Model file for the job. Use its own axes, mm. A direction names the side the tool comes from. Coordinates: 2 decimals unless noted, no trailing zeros. Loops run counter-clockwise (first coordinate to the right, second up) from the corner with the lowest first, then second, coordinate; pieces in that order, holes last. Notation, with made-up numbers: (57, -5.75) -> (90, -5.75) arc R17 cw to (90, 22.25) -> close; hole circle Ø6 at (-13.5, -22.5). An arc over 180 degrees is marked (long way). Use one line per item in the form item = value.
```python
from build123d import *

# Parameters (mm, degrees)
F0_W     = 48.26
F0_H     = 30.48
F0_W_2   = 45.72
F0_H_2   = 27.94
F1_DEPTH = 17.78
F2_DEPTH = 1.27
F3_R     = 7.62
F5_W     = 48.26
F5_H     = 17.78
F6_DEPTH = 1.27
F4_R     = 8.001
F4_R_2   = 7.62
F7_DEPTH = 12.1666


with BuildPart() as f1:
    # F0 (on Top) → F1 (new body)
    with BuildSketch(Plane.XY):
        with Locations((-40.818777, 0.441459)):
            Rectangle(F0_W, F0_H)
        with Locations((-40.818777, 0.441459)):
            Rectangle(F0_W_2, F0_H_2, mode=Mode.SUBTRACT)
    extrude(amount=F1_DEPTH)

    # F0 (on Top) → F2 (join)
    with BuildSketch(Plane.XY):
        with Locations((-40.818777, 0.441459)):
            Rectangle(F0_W_2, F0_H_2)
    extrude(amount=F2_DEPTH)

    # F3
    f3_edges = [f1.edges().sort_by_distance(p)[0] for p in [
        (-16.688777, 15.681459, 8.89),
        (-17.958777, 14.411459, 9.525),
    ]]
    fillet(f3_edges, radius=F3_R)

    # F5 (on face) → F6 (cut)
    with BuildSketch(Plane.XZ.offset(14.798541)):
        with Locations((-40.818777, 8.89)):
            Rectangle(F5_W, F5_H)
    extrude(amount=-F6_DEPTH, mode=Mode.SUBTRACT)

    # F4 (on face) → F7 (cut)
    with BuildSketch(Plane.XY.offset(1.27)):
        with Locations((-40.818777, 0.441459)):
            Circle(F4_R)
        with Locations((-26.086777, 6.283459)):
            Circle(F4_R_2)
        with Locations((-55.550777, -5.400541)):
            Circle(F4_R_2)
    extrude(amount=-F7_DEPTH, mode=Mode.SUBTRACT)


solid = f1.part
```
Q1. Which spindle directions (+Z, -Z, +X, -X, +Y, -Y) get a long thin tool onto all of the face, cutting with end or side? Do faces 1 (the face through (-41, 15, 17.78)), 2 (the face through (-17.959, -4, 9)). Say none if no direction does.
Result:
face_1 = +Z, +X, -X, +Y, -Y
face_2 = +Z, -Y
Q2. Mould opens along X. For faces 3 (the face through (-46, -6, 1.27)), 4 (the face through (-16.689, -3, 9)), 5 (the face through (-47, 8, 0)) say: released by +X, released by -X, zero draft, split by the parting line, or undercut.
Result:
face_3 = undercut
face_4 = released by +X
face_5 = zero draft
Q3. Pin check, flat tips, straight feed: pin 1 Ø8 at (x, y) = (-37, 7.5) entering from +Z; pin 2 Ø4 at (x, y) = (-29.5, 8) entering from -Z; pin 3 Ø4 at (x, z) = (-24.5, 11.5) entering from -Y. Stop position of each tip, or through.
Result:
pin_1 = 1.27
pin_2 = through
pin_3 = 13.76
Q4. Band-saw the part on A-A, the plane x = -53. Write the cut outline in (y, z), and give its area (3 significant figures).
Result:
outline = (-13.53, 0) -> (-12.58, 0) -> (-12.58, 1.27) -> (-13.53, 1.27) -> close; (1.78, 0) -> (15.68, 0) -> (15.68, 17.78) -> (14.41, 17.78) -> (14.41, 1.27) -> (1.78, 1.27) -> close
area = 39.8 mm2
Q5. Band-saw the part on B-B, the plane y = 10.75. Write the cut outline in (x, z).
Result:
outline = (-64.95, 0) -> (-32.26, 0) -> (-32.26, 1.27) -> (-63.68, 1.27) -> (-63.68, 17.78) -> (-64.95, 17.78) -> close; (-19.91, 0) -> (-17.18, 0) -> (-17.18, 17.78) -> (-19.07, 17.78) -> (-19.07, 1.27) -> (-19.91, 1.27) -> close
Q6. Wall check: line 1 along X through (y, z) = (-4, 7.5); line 2 along Y through (x, z) = (-37.5, 2.25); line 3 along Z through (x, y) = (-41.5, -12). Give the ranges that are in metal, low to high.
Result:
line_1 = -64.95 to -63.68, -17.96 to -16.69
line_2 = 14.41 to 15.68
line_3 = 0 to 1.27
Q7. Band-saw the part on D-D, the plane z = 8.75. Write the cut outline in (x, y), and give its area (3 significant figures).
Result:
outline = (-64.95, -13.53) -> (-63.68, -13.53) -> (-63.68, 14.41) -> (-25.58, 14.41) arc R7.62 cw to (-17.96, 6.79) -> (-17.96, -13.53) -> (-16.69, -13.53) -> (-16.69, 8.06) arc R7.62 ccw to (-24.31, 15.68) -> (-64.95, 15.68) -> close
area = 132 mm2
Q8. Band-saw the part on C-C, the plane y = 3. Write the cut outline in (x, z), and give its area (3 significant figures).
Result:
outline = (-64.95, 0) -> (-48.4, 0) -> (-48.4, 1.27) -> (-63.68, 1.27) -> (-63.68, 17.78) -> (-64.95, 17.78) -> close; (-33.24, 0) -> (-32.96, 0) -> (-32.96, 1.27) -> (-33.24, 1.27) -> close; (-19.21, 0) -> (-16.69, 0) -> (-16.69, 17.78) -> (-17.96, 17.78) -> (-17.96, 1.27) -> (-19.21, 1.27) -> close
area = 66.5 mm2
